from build123d import *

# Parameters (mm, degrees)
F0_R         = 19.8
F1_DEPTH     = 5
F2_R         = 16.8
F2_R_2       = 16
F3_DEPTH     = 1.8
F6_DEPTH     = 3
F7_T4_DEPTH  = 62.0556939075
F7_S5_R      = 19.8
F7_T6_DEPTH  = 33
F7_T10_DEPTH = 62.0556939075
F7_S11_R     = 19.8
F7_T12_DEPTH = 33


# Not quite as in the source:
# - a fillet or chamfer that OpenCascade refuses, or shapes differently, is made with other operations: its cross-section is extruded or revolved along the edge and cut away or added


with BuildPart() as f1:
    # F0 (on Top) → F1 (new body)
    with BuildSketch(Plane.XY):
        Circle(F0_R)
    extrude(amount=F1_DEPTH)

    # F2 (on face) → F3 (join)
    with BuildSketch(Plane.XY.offset(5)):
        Circle(F2_R)
        Circle(F2_R_2, mode=Mode.SUBTRACT)
    extrude(amount=F3_DEPTH)

    # F4: chamfer of 4 on 1 edges, made by hand


with BuildPart() as f4_tool2:
    # F4_s3 → F4_t4 (revolve)
    with BuildSketch(Plane.XZ):
        Polygon((16, 9), (12, 5), (16, 5), align=None)
    revolve(axis=Axis((0, 0, 5), (0, 0, 1)))

    split(bisect_by=Plane.XY.offset(6.8), keep=Keep.BOTTOM)


with BuildPart() as f1_1:
    add(f1.part)

    # F4_t1: union F4_tool2
    add(f4_tool2.part)

    # F5 (on face) → F6 (cut)
    with BuildSketch(Plane(origin=(0, 0, 0), x_dir=(1, 0, 0), z_dir=(0, 0, -1))):
        with BuildLine():
            Line((-3, 19.5714077164), (-3, -19.5714077164))
            ThreePointArc((-3, -19.5714077164), (0, -19.8), (3, -19.5714077164))
            Line((3, -19.5714077164), (3, 19.5714077164))
            ThreePointArc((3, 19.5714077164), (0, 19.8), (-3, 19.5714077164))
        make_face()
    extrude(amount=-F6_DEPTH, mode=Mode.SUBTRACT)

    # F7: fillet of radius 5 on 2 edges, made by hand


with BuildPart() as f7_tool2:
    # F7_s3 → F7_t4 (new body)
    with BuildSketch(Plane.XZ.offset(-31.0278469537)):
        with BuildLine():
            ThreePointArc((3, 0), (1.1560370926, 2.1833001327), (-1.582575695, 3))
            Line((-1.582575695, 3), (3, 3))
            Line((3, 3), (3, 0))
        make_face()
    extrude(amount=F7_T4_DEPTH)

    # F7_s5 → F7_t6 (intersect, symmetric)
    with BuildSketch(Plane.XY.offset(1.5)):
        Circle(F7_S5_R)
    extrude(amount=F7_T6_DEPTH, both=True, mode=Mode.INTERSECT)


with BuildPart() as f1_2:
    add(f1_1.part)

    # F7_t1: union F7_tool2
    add(f7_tool2.part)


with BuildPart() as f7_tool8:
    # F7_s9 → F7_t10 (new body)
    with BuildSketch(Plane.XZ.offset(31.0278469537)):
        with BuildLine():
            ThreePointArc((1.582575695, 3), (-1.1560370926, 2.1833001327), (-3, 0))
            Line((-3, 0), (-3, 3))
            Line((-3, 3), (1.582575695, 3))
        make_face()
    extrude(amount=-F7_T10_DEPTH)

    # F7_s11 → F7_t12 (intersect, symmetric)
    with BuildSketch(Plane.XY.offset(1.5)):
        Circle(F7_S11_R)
    extrude(amount=F7_T12_DEPTH, both=True, mode=Mode.INTERSECT)


with BuildPart() as f1_3:
    add(f1_2.part)

    # F7_t7: union F7_tool8
    add(f7_tool8.part)


solid = f1_3.part
The listing builds one solid part. Answer for the finished solid, in the listing's coordinates (mm). A direction names the side the tool comes from. Give positions to 0.01 mm unless a question says otherwise; leave off trailing zeros. Order: outer loops, then holes, each group sorted by start corner. A loop starts at its lowest first (then second) coordinate and runs counter-clockwise, first axis right, second up. Notation, with made-up numbers: (20, 18) - (70, 18) arc R22 cw to (70, 32) - close; hole circle Ø5 at (66, -37). An arc over 180 degrees is marked (long way). One line per item, written item: value. Start each with the question number.
1) Find the intervals of material crossed by L1, parallel to X at y = 12, z = 0.5; L2, parallel to Z at x = 9, y = -16.5; L3, parallel to X at y = 3, z = 1.5, in increasing order.
2) A cutting plane is placed at A-A on z = 6. Give the vertices of the cut face in (x, y), then the cut area to 3 significant figures.
3) A cutting plane is placed at C-C on z = 1.5. Give the vertices of the cut face in (x, y), then the cut area to 3 significant figures.
4) Given pin 1 Ø12 at (x, y) = (-2.5, 4) entering from +Z; pin 2 Ø1.5 at (y, z) = (4.5, 3.5) entering from +X, each flat-ended and moving along its own axis, determine where each tip first touches the part or whether it passes through.
5) A cutting plane is placed at B-B on y = 0. Give the vertices of the cut face in (x, z), then the cut area to 3 significant figures.
6) The mould has two halves that part along X. Classify faces 4 (the face through (16.024, 5.046, 5.887)), 5 (the face through (-1.77, -0.28, 1.71)), 6 (the face through (9, 0, 0)): released by +X, released by -X, zero draft, split by the parting line, or undercut.
7) A tool of negligible diameter and unlimited length cuts with its end or side. For faces 1 (the face through (-9, -15, 5)), 2 (the face through (-10, 0, 0)), 3 (the face through (1.813, 0.277, 1.67)), from which of +Z, -Z, +X, -X, +Y, -Y can it reach the whole face along a straight path? Write none if from no direction.
Answer sheet:
1. L1: x = -15.75 to -2.75, 2.75 to 15.75
1. L2: z = 0 to 5
1. L3: x = -19.57 to -1.99, 1.99 to 19.57
2. outline: circle Ø33.6 at (0, 0); hole circle Ø26 at (0, 0)
2. area: 356 mm2
3. outline: (-1.99, -19.7) - (-1.99, 19.7) arc R19.8 ccw to start; (1.99, -19.7) arc R19.8 ccw to (1.99, 19.7) - close
3. area: 1,070 mm2
4. pin 1: stops at z = 5
4. pin 2: stops at x = 19.44
5. outline: (-19.8, 0) - (-3, 0) arc R5 cw to (0, 2.74) arc R5 cw to (3, 0) - (19.8, 0) - (19.8, 5) - (16.8, 5) - (16.8, 6.8) - (13.8, 6.8) - (12, 5) - (-12, 5) - (-13.8, 6.8) - (-16.8, 6.8) - (-16.8, 5) - (-19.8, 5) - close
5. area: 201 mm2
6. face 4: split by the parting line
6. face 5: undercut
6. face 6: zero draft
7. face 1: +Z
7. face 2: -Z, +X, -X, +Y, -Y
7. face 3: -Z, +Y, -Y
